Part model, mm, in its own coordinate system. A direction names the side the tool comes from. Round coordinates to 2 decimals unless told otherwise and drop trailing zeros. Loops run counter-clockwise (first coordinate to the right, second up) from the corner with the lowest first, then second, coordinate; pieces in that order, holes last.
1) Band-saw the part on C-C, the plane z = -5.3. Write the cut outline in (x, y).
2) Band-saw the part on D-D, the plane y = 8.25. Write the cut outline in (x, z), then the cut area to 3 significant figures.
3) Band-saw the part on A-A, the plane x = 6.25. Write the cut outline in (y, z), then the cut area to 3 significant figures.
4) Band-saw the part on B-B, the plane y = 1.5. Write the cut outline in (x, z).
5) Probe line 1 (X direction, y = 0.9, z = -5.3); line 2 (Z direction, x = 39, y = 3.25); line 3 (Y direction, x = 42.5, z = -7). List the from-to ranges inside material, lowest first.
6) Mould opens along X. For faces 1 (the flat face through (5, 2, -7)), 2 (the flat face through (50, 3, -1)), 3 (the flat face through (37.5, 1, -5)) say: +X half, -X half, draft (parallel to the pull), parting line (faces both ways), or undercut.
7) Drop flat-ended pins along their axis: P1, Ø3, axis at x = 21, y = 3.5, coming from the -Z side; P2, Ø4.5, axis at x = 6.25, z = -5.3, coming from the +Y side. Give the stop position or say it passes through.
8) 3-axis set-ups, long thin cutter, end or side, ignore diameter. For faces 4 (the flat face through (12.5, 1, -5)), 5 (the flat face through (45, 2, -7)), 6 (the cylindrical face through (45.535, 1.014, -5.534)): which of +Z, -Z, +X, -X, +Y, -Y reach the whole face in a straight line?
from build123d import *

# Parameters (mm, degrees)
SKETCH1_W           = 50
SKETCH1_H           = 8.6
BOSS_EXTRUDE2_DEPTH = 2
SKETCH3_W           = 50
SKETCH3_H           = 2
BOSS_EXTRUDE3_DEPTH = 8
SKETCH4_W           = 25
SKETCH4_H           = 6.6
CUT_EXTRUDE1_DEPTH  = 8
SKETCH5_W           = 25
SKETCH5_H           = 2
CUT_EXTRUDE2_DEPTH  = 2
SKETCH6_R           = 1.8
CUT_EXTRUDE3_DEPTH  = 2
BOSS_EXTRUDE4_DEPTH = 0.5
SKETCH8_W           = 25
SKETCH8_H           = 2
BOSS_EXTRUDE5_DEPTH = 2.5


with BuildPart() as part:
    # Sketch1 → Boss-Extrude2 (new body)
    with BuildSketch(Plane(origin=(0, 0, 0), x_dir=(1, 0, 0), z_dir=(0, 1, 0))):
        with Locations((25, 4.3)):
            Rectangle(SKETCH1_W, SKETCH1_H)
    extrude(amount=BOSS_EXTRUDE2_DEPTH)

    # Sketch3 → Boss-Extrude3 (add)
    with BuildSketch(Plane(origin=(0, 2, 0), x_dir=(1, 0, 0), z_dir=(0, 1, 0))):
        with Locations((25, 1)):
            Rectangle(SKETCH3_W, SKETCH3_H)
    extrude(amount=BOSS_EXTRUDE3_DEPTH)

    # Sketch4 → Cut-Extrude1 (cut)
    with BuildSketch(Plane(origin=(0, 2, 0), x_dir=(1, 0, 0), z_dir=(0, 1, 0))):
        with Locations((25, 5.3)):
            Rectangle(SKETCH4_W, SKETCH4_H)
    extrude(amount=-CUT_EXTRUDE1_DEPTH, mode=Mode.SUBTRACT)

    # Sketch5 → Cut-Extrude2 (cut)
    with BuildSketch(Plane(origin=(0, 0, -2), x_dir=(-1, 0, 0), z_dir=(0, 0, -1))):
        with Locations((-25, 1)):
            Rectangle(SKETCH5_W, SKETCH5_H)
    extrude(amount=-CUT_EXTRUDE2_DEPTH, mode=Mode.SUBTRACT)

    # Sketch6 → Cut-Extrude3 (cut)
    with BuildSketch(Plane(origin=(0, 2, 0), x_dir=(1, 0, 0), z_dir=(0, 1, 0))):
        with Locations(Location((43.75, 5.3, 0), (0, 0, 270))):
            Circle(SKETCH6_R)
        with Locations(Location((6.25, 5.3, 0), (0, 0, 270))):
            Circle(SKETCH6_R)
    extrude(amount=-CUT_EXTRUDE3_DEPTH, mode=Mode.SUBTRACT)

    # Sketch7 → Boss-Extrude4 (add)
    with BuildSketch(Plane.XY):
        Polygon((12.5, 0), (0, 0), (0, 10), (50, 10), (50, 0), (37.5, 0), (37.5, 2), (12.5, 2), align=None)
    extrude(amount=BOSS_EXTRUDE4_DEPTH)

    # Sketch8 → Boss-Extrude5 (add)
    with BuildSketch(Plane.XY.offset(0.5)):
        with Locations((25, 1)):
            Rectangle(SKETCH8_W, SKETCH8_H)
    extrude(amount=-BOSS_EXTRUDE5_DEPTH)


solid = part.part
Reported:
1. outline: (0, 0) - (4.45, 0) - (4.45, 2) - (0, 2) - close; (8.05, 0) - (12.5, 0) - (12.5, 2) - (8.05, 2) - close; (37.5, 0) - (41.95, 0) - (41.95, 2) - (37.5, 2) - close; (45.55, 0) - (50, 0) - (50, 2) - (45.55, 2) - close
2. outline: (0, -2) - (50, -2) - (50, 0.5) - (0, 0.5) - close
2. area: 125 mm2
3. outline: (0, -8.6) - (2, -8.6) - (2, -7.1) - (0, -7.1) - close; (0, -3.5) - (2, -3.5) - (2, -2) - (10, -2) - (10, 0.5) - (0, 0.5) - close
3. area: 31.0 mm2
4. outline: (0, -8.6) - (12.5, -8.6) - (12.5, -2) - (37.5, -2) - (37.5, -8.6) - (50, -8.6) - (50, 0.5) - (0, 0.5) - close; hole circle Ø3.6 at (6.25, -5.3); hole circle Ø3.6 at (43.75, -5.3)
5. line 1: x = 0 to 4.45, 8.05 to 12.5, 37.5 to 41.95, 45.55 to 50
5. line 2: z = -2 to 0.5
5. line 3: y = 0 to 2
6. face 1: draft
6. face 2: +X half
6. face 3: undercut
7. P1: stops at z = -2
7. P2: stops at y = 2
8. face 4: -Z, +Y, -Y
8. face 5: -Z, +X, -X, +Y
8. face 6: +Y, -Y
